Can you work these out from the model? Positions are in its coordinate system, mm. Face numbers are marked on the shaded views. A direction names the side the tool comes from. Give positions to 0.01 mm unless a question says otherwise; leave off trailing zeros. Loops run counter-clockwise (first coordinate to the right, second up) from the corner with the lowest first, then second, coordinate; pieces in that order, holes last. Notation, with made-up numbers: M 75,57 L 103,57 A26 ccw 103,91 Z; hole C -40,87.5 d9. An arc over 180 degrees is marked long. Answer as a JSON object with one key per item and string values.
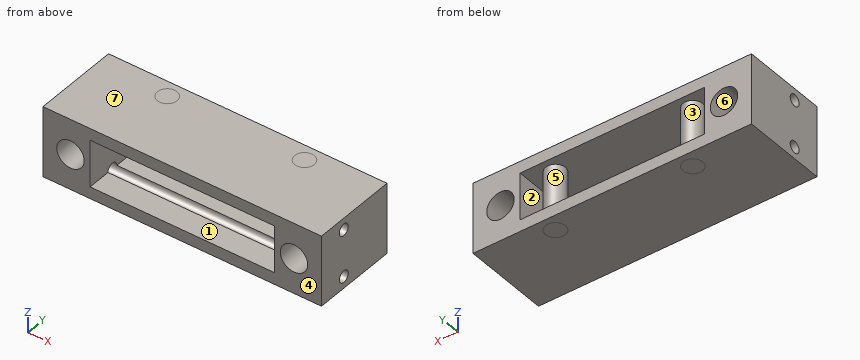
Autodesk Inventor part; units mm, degrees
ref_plane "YZ Plane" through (0, 0, 0) normal (1, 0, 0) x (0, 1, 0)
ref_plane "XZ Plane" through (0, 0, 0) normal (0, 1, 0) x (-1, 0, 0)
ref_plane "XY Plane" through (0, 0, 0) normal (0, 0, 1) x (1, 0, 0)
sketch "Esquisse1" plane through (0, 0, 0) normal (0, 1, 0) x (-1, 0, 0)
  circle A0 centre (-28.5, 0) radius 3.5
  circle A1 centre (28.5, 0) radius 3.5
  line L0 (-35.5, 9) -> (35.5, 9)
  line L1 (35.5, 9) -> (35.5, -9)
  line L2 (35.5, -9) -> (-35.5, -9)
  line L3 (-35.5, -9) -> (-35.5, 9)
  line L4 (-28.5, 0) -> (28.5, 0)
  point P0 (0, 0)
  dimension "d0" = 7
  dimension "d1" = 7
  dimension "d2" = 28.5
  dimension "d3" = 28.5
  dimension "d4" = 18
  dimension "d5" = 9
  dimension "d6" = 7
  dimension "d7" = 7
extrude "Extrusion1" add sketch "Esquisse1" along normal blind 22
sketch "Esquisse2" plane through (0, 22, 0) normal (0, 1, 0) x (1, 0, 0)
  circle A0 centre (-28.5, 0) radius 3.5
  circle A1 centre (28.5, 0) radius 3.5
  line L0 (-23.5, 6) -> (23.5, 6)
  line L1 (23.5, 6) -> (23.5, -6)
  line L2 (23.5, -6) -> (-23.5, -6)
  line L3 (-23.5, -6) -> (-23.5, 6)
  point P0 (0, 0)
  dimension "d10" = 12
  dimension "d11" = 6
  dimension "d12" = 5
  dimension "d13" = 5
extrude "Extrusion2" cut sketch "Esquisse2" against normal through all contours L0 L1 L2 L3
sketch "Esquisse3" plane through (-35.5, 0, 9) normal (0, 0, 1) x (1, 0, 0)
  line L0 (71, 0) -> (0, 0)
  line L1 (71, 0) -> (71, 22)
  line L2 (0, 22) -> (71, 22)
  line L3 (0, 0) -> (0, 22)
  line L4 (14, 22) -> (57, 22)
  line L5 (57, 22) -> (57, 0)
  line L6 (57, 0) -> (14, 0)
  line L7 (14, 0) -> (14, 22)
  line L8 (14, 22) -> (22, 22)
  line L9 (22, 22) -> (22, 14)
  line L10 (22, 14) -> (14, 14)
  line L11 (14, 14) -> (14, 22)
  line L12 (57, 22) -> (49, 22)
  line L13 (49, 22) -> (49, 14)
  line L14 (49, 14) -> (57, 14)
  line L15 (57, 14) -> (57, 22)
  line L16 (14, 22) -> (22, 14)
  line L17 (22, 22) -> (14, 14)
  line L18 (49, 14) -> (57, 22)
  line L19 (49, 22) -> (57, 14)
  circle A0 centre (18, 18) radius 2.5
  circle A1 centre (53, 18) radius 2.5
  point P0 (35.5, 0)
  dimension "d16" = 14
  dimension "d17" = 14
  dimension "d18" = 8
  dimension "d19" = 8
  dimension "d20" = 8
  dimension "d21" = 8
  dimension "d22" = 5
  dimension "d23" = 5
sketch "Esquisse3 outline for Extrusion3" plane through (-35.5, 0, 9) normal (0, 0, 1) x (1, 0, 0)
  circle A0 centre (18, 18) radius 2.5
  circle A1 centre (53, 18) radius 2.5
extrude "Extrusion3" add sketch "Esquisse3 outline for Extrusion3" along normal through all both and the other way through all
sketch "Esquisse4" plane through (35.5, 0, 9) normal (1, 0, 0) x (0, 0, -1)
  line L0 (18, 0) -> (0, 0)
  line L1 (0, 22) -> (18, 22)
  line L2 (6, 22) -> (12, 22)
  line L3 (12, 22) -> (12, 0)
  line L4 (12, 0) -> (6, 0)
  line L5 (6, 0) -> (6, 22)
  circle A0 centre (3, 7.5) radius 1.5
  circle A1 centre (15, 7.5) radius 1.5
  line L6 (18, 0) -> (18, 22)
  line L7 (0, 0) -> (6, 0)
  line L8 (6, 0) -> (6, 15)
  line L9 (6, 15) -> (0, 15)
  line L10 (0, 15) -> (0, 0)
  line L11 (12, 0) -> (18, 0)
  line L12 (18, 0) -> (18, 15)
  line L13 (18, 15) -> (12, 15)
  line L14 (12, 15) -> (12, 0)
  line L15 (0, 15) -> (6, 0)
  line L16 (6, 15) -> (0, 0)
  line L17 (12, 15) -> (18, 0)
  line L18 (18, 15) -> (12, 0)
  point P0 (9, 0)
  point P1 (3, 7.5)
  point P2 (15, 7.5)
  dimension "d26" = 6
  dimension "d27" = 3
  dimension "d28" = 3
  dimension "d29" = 3
  dimension "d32" = 15
extrude "Extrusion4" cut sketch "Esquisse4" against normal through all contours L17 L18 A1 | A1 L18 L17 | A1 L17 L18 | L18 L17 A1 | L15 L16 A0 | A0 L16 L15 | A0 L15 L16 | L16 L15 A0
equation "\"d5\" = 0.5 * d4"
equation "\"d17\" = d16"
properties part number "tendeur_base"
1) Please list where these lines run through material, in increasing order: line 1 along Z through (x, y) = (22, 20.5); line 2 along Z through (x, y) = (-28.5, 5.75); line 3 along X through (y, z) = (17.25, -3.75). Write a range as from..to.
Answer list:
{"line 1": "-9..-6, 6..9", "line 2": "-9..-3.5, 3.5..9", "line 3": "-35.5..-23.5, -19.88..-15.12, 15.12..19.88, 23.5..35.5"}
2) For the marked faces 1, 2 and 3, which set-ups out of +Z, -Z, +X, -X, +Y, -Y let a thin tool reach every point of the face, with its end or its side?
Answer list:
{"face 1": "-Y", "face 2": "+Y, -Y", "face 3": "none"}
3) If we mould it in two halves opening along Z, with no side actions, what happens to the marked faces 4, 5, 6 and 7? For each: +Z half, -Z half, draft (parallel to the pull), parting line (faces both ways), or undercut.
Answer list:
{"face 4": "draft", "face 5": "undercut", "face 6": "undercut", "face 7": "+Z half"}
4) Suppose I cut it at C-C, the plane y = 7.5. Write out the boundary of the cut face in (x, z).
Answer list:
{"outline": "M -35.5,-9 L 35.5,-9 L 35.5,-7.5 L -35.5,-7.5 Z; M -35.5,-4.5 L -23.5,-4.5 L -23.5,4.5 L -35.5,4.5 Z; M -35.5,7.5 L 35.5,7.5 L 35.5,9 L -35.5,9 Z; M 23.5,-4.5 L 35.5,-4.5 L 35.5,4.5 L 23.5,4.5 Z; hole C -28.5,0 d7; hole C 28.5,0 d7"}
5) Suppose I cut it at D-D, the plane y = 18. Give the number of separate pieces and of enclosed holes in the cut face, and give its area (3 significant figures).
Answer list:
{"separate pieces": "1", "enclosed holes": "5", "area": "757 mm^2"}
6) Suppose I cut it at A-A, the plane x = -28.5. Write out the boundary of the cut face in (y, z), and give its area (3 significant figures).
Answer list:
{"outline": "M 0,-9 L 22,-9 L 22,-3.5 L 0,-3.5 Z; M 0,3.5 L 22,3.5 L 22,9 L 0,9 Z; hole C 7.5,-6 d3; hole C 7.5,6 d3", "area": "228 mm^2"}
7) Suppose I cut it at B-B, the plane z = 0. Write out the boundary of the cut face in (x, y).
Answer list:
{"outline": "M -35.5,0 L -32,0 L -32,22 L -35.5,22 Z; M -25,0 L -23.5,0 L -23.5,22 L -25,22 Z; C -17.5,18 d5; C 17.5,18 d5; M 23.5,0 L 25,0 L 25,22 L 23.5,22 Z; M 32,0 L 35.5,0 L 35.5,22 L 32,22 Z"}
